For this review, take the finished solid that the model builds, in its own axes (mm). Give positions to 0.01 mm unless a question says otherwise; leave off trailing zeros. Order: outer loops, then holes, each group sorted by start corner. A loop starts at its lowest first (then second) coordinate and runs counter-clockwise, first axis right, second up. Notation, with made-up numbers: (56.25, 62) -> (87.25, 62) arc R12 ccw to (87.25, 71) -> close; hole circle Ø11 at (79, 87). An arc over 180 degrees is marked (long way). Return JSON: item names as keys, results as strings. Group by question number.
1) Add section A-A (z = 47.5). Give the boundary of the cut face in (x, y).
2) To check wall thickness, follow line 1 along X through (y, z) = (0.8, 35); line 2 along X through (y, z) = (1.6, -47.5); line 3 along Z through (x, y) = (-4, 1.25). State the ranges of each line that lie inside material, in increasing order.
3) Add section B-B (x = 0). State how many separate pieces and enclosed holes the cut face has, then the cut area to 3 significant figures.
4) Add section D-D (y = 1.95). Give the boundary of the cut face in (x, z), then the cut area to 3 significant figures.
from build123d import *

# Parameters (mm, degrees)
SKETCH_1_W          = 57
SKETCH_1_H          = 99.6
SKETCH_1_R          = 1.7
EXTRUDE_1_DEPTH     = 3
SKETCH_2_W          = 40
SKETCH_2_H          = 10
CUT_EXTRUDE_1_DEPTH = 3
CHAMFER_1_SIZE      = 3


with BuildPart() as part:
    # 草图1 → 凸台-拉伸1 (new body)
    with BuildSketch(Plane(origin=(0, 0, 0), x_dir=(1, 0, 0), z_dir=(0, 1, 0))):
        Rectangle(SKETCH_1_W, SKETCH_1_H)
        with Locations(Location((0, 47.5, 0), (0, 0, 270))):
            Circle(SKETCH_1_R, mode=Mode.SUBTRACT)
        with Locations(Location((0, -47.5, 0), (0, 0, 270))):
            Circle(SKETCH_1_R, mode=Mode.SUBTRACT)
    extrude(amount=EXTRUDE_1_DEPTH)

    # 草图2 → 切除-拉伸1 (cut)
    with BuildSketch(Plane(origin=(0, 3, 0), x_dir=(1, 0, 0), z_dir=(0, 1, 0))):
        with Locations((0, 35)):
            Rectangle(SKETCH_2_W, SKETCH_2_H)
        with Locations((0, -35)):
            Rectangle(SKETCH_2_W, SKETCH_2_H)
    extrude(amount=-CUT_EXTRUDE_1_DEPTH, mode=Mode.SUBTRACT)

    # 倒角1
    chamfer_1_edges = [part.edges().sort_by_distance(p)[0] for p in [
        (0, 3, 40),
        (0, 3, -40),
    ]]
    chamfer(chamfer_1_edges, length=CHAMFER_1_SIZE - 0.0001)  # a hair under: the kernel refuses the full size


solid = part.part
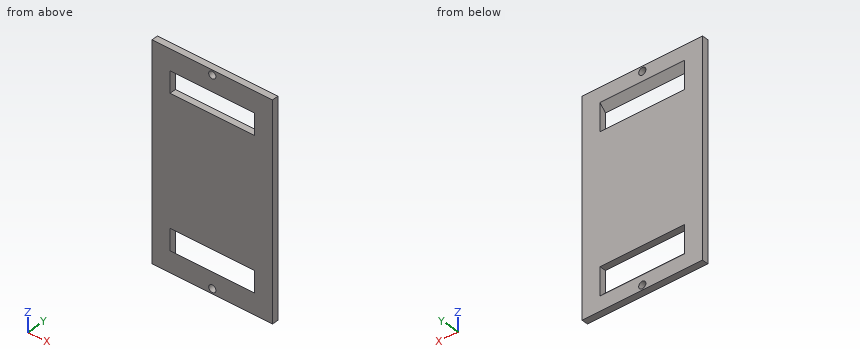
Evaluation:
{
 "1": {"outline": "(-28.5, 0) -> (-1.7, 0) -> (-1.7, 3) -> (-28.5, 3) -> close; (1.7, 0) -> (28.5, 0) -> (28.5, 3) -> (1.7, 3) -> close"},
 "2": {"line 1": "-28.5 to -20, 20 to 28.5", "line 2": "-28.5 to -1.7, 1.7 to 28.5", "line 3": "-49.8 to -41.25, -30 to 30, 41.25 to 49.8"},
 "3": {"separate pieces": "5", "enclosed holes": "0", "area": "209 mm^2"},
 "4": {"outline": "(-28.5, -49.8) -> (28.5, -49.8) -> (28.5, 49.8) -> (-28.5, 49.8) -> close; hole (-20, -41.95) -> (20, -41.95) -> (20, -30) -> (-20, -30) -> close; hole (-20, 30) -> (20, 30) -> (20, 41.95) -> (-20, 41.95) -> close; hole circle Ø3.4 at (0, -47.5); hole circle Ø3.4 at (0, 47.5)", "area": "4,700 mm^2"}
}
